Geometry: final body of the model. Coordinates: model frame, mm. A direction names the side the tool comes from. Give positions to 0.01 mm unless a question says otherwise; leave off trailing zeros. Loops run counter-clockwise (first coordinate to the right, second up) from the corner with the lowest first, then second, coordinate; pieces in that order, holes last.
1. Section C-C, the plane y = 60. Output: boundary loops of the cut face in (x, z), then the cut area to 3 significant figures.
2. First-contact query: P1, Ø11, axis at x = 507.5, z = 216, coming from the +Y side; P2, Ø11, axis at x = 142.5, y = 24, coming from the -Z side; P3, Ø6, axis at y = 74.5, z = 11, coming from the +X side; P4, Ø4, axis at x = 512.5, y = 20.5, coming from the +Z side. Flat tips, straight axial feed; report the tip coordinate or a pass-through.
3. Material intervals for line 1 along X through (y, z) = (27, 520); line 2 along Z through (x, y) = (262, 25), sorted ascending.
4. Access query for faces 1 (the face through (-60, 27.996, 281)), 2 (the face through (-60, 80, 17)), 3 (the face through (219, 21, 573)), 4 (the face through (510, 13.996, 301)). Directions: +Z, -Z, +X, -X, +Y, -Y. A direction counts if a zero-diameter tool reaches every point of the face in a straight line with its end or side. Return the directions, or none.
5. Section B-B, the plane x = 103. Output: boundary loops of the cut face in (y, z), then the cut area to 3 significant figures.
6. Section A-A, the plane z = 79.5. Output: boundary loops of the cut face in (x, y).
7. Draft query along Y for faces 5 (the face through (510, 27.996, 301)), 6 (the face through (-52.505, 80, 10)). Return one class per face: +Y half, -Y half, draft (parallel to the pull), parting line (faces both ways), or undercut.
from build123d import *

# Parameters (mm, degrees)
SKETCH_1_W      = 20
SKETCH_1_H      = 20
SKETCH_1_W_2    = 14
SKETCH_1_H_2    = 14
EXTRUDE_1_DEPTH = 570
SKETCH_2_W      = 20
SKETCH_2_H      = 20
SKETCH_2_W_2    = 14
SKETCH_2_H_2    = 14
EXTRUDE_2_DEPTH = 100
SKETCH_5_W      = 20
SKETCH_5_H      = 20
SKETCH_5_W_2    = 14
SKETCH_5_H_2    = 14
EXTRUDE_3_DEPTH = 570
SKETCH_6_W      = 20
SKETCH_6_H      = 20
SKETCH_6_W_2    = 14
SKETCH_6_H_2    = 14
EXTRUDE_4_DEPTH = 570
SKETCH_7_W      = 20
SKETCH_7_H      = 20
SKETCH_7_W_2    = 14
SKETCH_7_H_2    = 14
EXTRUDE_5_DEPTH = 570


with BuildPart() as part:
    # 草图1 → 凸台-拉伸1 (new body)
    with BuildSketch(Plane.XY):
        with Locations((-59.504950495, 20.995577113)):
            Rectangle(SKETCH_1_W, SKETCH_1_H)
        with Locations((-59.504950495, 20.995577113)):
            Rectangle(SKETCH_1_W_2, SKETCH_1_H_2, mode=Mode.SUBTRACT)
    extrude(amount=EXTRUDE_1_DEPTH)

    # 草图2 → 凸台-拉伸2 (add)
    with BuildSketch(Plane(origin=(0, 30.995577113, 0), x_dir=(1, 0, 0), z_dir=(0, 1, 0))):
        with Locations((-59.504950495, -10)):
            Rectangle(SKETCH_2_W, SKETCH_2_H)
        with Locations((-59.504950495, -10)):
            Rectangle(SKETCH_2_W_2, SKETCH_2_H_2, mode=Mode.SUBTRACT)
    extrude(amount=EXTRUDE_2_DEPTH)

    # 草图5 → 凸台-拉伸3 (add)
    with BuildSketch(Plane(origin=(-49.504950495, 0, 0), x_dir=(0, 0, -1), z_dir=(1, 0, 0))):
        with Locations((-10, 20.995577113)):
            Rectangle(SKETCH_5_W, SKETCH_5_H)
        with Locations((-10, 20.995577113)):
            Rectangle(SKETCH_5_W_2, SKETCH_5_H_2, mode=Mode.SUBTRACT)
    extrude(amount=EXTRUDE_3_DEPTH)

    # 草图6 → 凸台-拉伸4 (add)
    with BuildSketch(Plane.XY.offset(20)):
        with Locations((510.495049505, 20.995577113)):
            Rectangle(SKETCH_6_W, SKETCH_6_H)
        with Locations((510.495049505, 20.995577113)):
            Rectangle(SKETCH_6_W_2, SKETCH_6_H_2, mode=Mode.SUBTRACT)
    extrude(amount=EXTRUDE_4_DEPTH)

    # 草图7 → 凸台-拉伸5 (add)
    with BuildSketch(Plane.ZY.offset(-500.495049505)):
        with Locations((580, 20.995577113)):
            Rectangle(SKETCH_7_W, SKETCH_7_H)
        with Locations((580, 20.995577113)):
            Rectangle(SKETCH_7_W_2, SKETCH_7_H_2, mode=Mode.SUBTRACT)
    extrude(amount=EXTRUDE_5_DEPTH)


solid = part.part
Answers below:
1. outline: (-69.5, 0) - (-49.5, 0) - (-49.5, 20) - (-69.5, 20) - close; hole (-66.5, 3) - (-52.5, 3) - (-52.5, 17) - (-66.5, 17) - close
1. area: 204 mm2
2. P1: stops at y = 31
2. P2: stops at z = 0
2. P3: stops at x = -49.5
2. P4: stops at z = 20
3. line 1: x = -69.5 to -66.5, -52.5 to -49.5, 500.5 to 503.5, 517.5 to 520.5
3. line 2: z = 0 to 3, 17 to 20, 570 to 573, 587 to 590
4. face 1: -Z
4. face 2: +Y
4. face 3: -X
4. face 4: +Z
5. outline: (11, 0) - (31, 0) - (31, 20) - (11, 20) - close; (11, 570) - (31, 570) - (31, 590) - (11, 590) - close; hole (14, 3) - (28, 3) - (28, 17) - (14, 17) - close; hole (14, 573) - (28, 573) - (28, 587) - (14, 587) - close
5. area: 408 mm2
6. outline: (-69.5, 11) - (-49.5, 11) - (-49.5, 31) - (-69.5, 31) - close; (500.5, 11) - (520.5, 11) - (520.5, 31) - (500.5, 31) - close; hole (-66.5, 14) - (-52.5, 14) - (-52.5, 28) - (-66.5, 28) - close; hole (503.5, 14) - (517.5, 14) - (517.5, 28) - (503.5, 28) - close
7. face 5: undercut
7. face 6: draft
